Check sheet for the modelled part. Datum: model origin and axes. Units: mm. A direction names the side the tool comes from. Coordinates: 2 decimals unless noted, no trailing zeros. Loops run counter-clockwise (first coordinate to the right, second up) from the corner with the lowest first, then second, coordinate; pieces in that order, holes last. Notation, with made-up numbers: M 22,21.25 L 76,21.25 A35 ccw 76,57.25 Z; hole C 74.5,19.5 d5. An arc over 180 degrees is marked long. Return JSON: item names as keys, results as strings.
from build123d import *

# Parameters (mm, degrees)
F0_W     = 914.4
F0_H     = 914.4
F0_W_2   = 254
F0_H_2   = 889
F0_W_3   = 38.1
F1_DEPTH = 25.4


with BuildPart() as f1:
    # F0 (on Top) → F1 (new body)
    with BuildSketch(Plane.XY):
        with Locations((34.239113, 103.026486)):
            Rectangle(F0_W, F0_H)
        with Locations((-283.260887, 103.026486)):
            Rectangle(F0_W_2, F0_H_2, mode=Mode.SUBTRACT)
        with Locations((-124.510887, 103.026486)):
            Rectangle(F0_W_3, F0_H_2, mode=Mode.SUBTRACT)
        with Locations((34.239113, 103.026486)):
            Rectangle(F0_W_2, F0_H_2, mode=Mode.SUBTRACT)
        with Locations((192.989113, 103.026486)):
            Rectangle(F0_W_3, F0_H_2, mode=Mode.SUBTRACT)
        with Locations((351.739113, 103.026486)):
            Rectangle(F0_W_2, F0_H_2, mode=Mode.SUBTRACT)
    extrude(amount=F1_DEPTH)


solid = f1.part
1) Section check A-A on x = -79. Record the cut outline in (y, z), then the cut area to 3 significant figures.
Answers:
{"outline": "M -354.17,0 L -341.47,0 L -341.47,25.4 L -354.17,25.4 Z; M 547.53,0 L 560.23,0 L 560.23,25.4 L 547.53,25.4 Z", "area": "645 mm²"}
2) Set-up check for faces 5 (the face through (32, -341.474, 13)), 6 (the face through (-103, 105, 0)): record each of +Z, -Z, +X, -X, +Y, -Y from which the full face is reachable in a straight line by a thin tool's end or side.
Answers:
{"face 5": "+Z, -Z", "face 6": "-Z, +X, -X, +Y, -Y"}
3) Draft check along Y on faces 1 (the face through (-156.261, 97, 13)), 2 (the face through (28, -354.174, 13)), 3 (the face through (-422.961, 97, 13)), 4 (the face through (-143.561, 97, 13)). Enter one of: +Y half, -Y half, draft (parallel to the pull), parting line (faces both ways), or undercut.
Answers:
{"face 1": "undercut", "face 2": "-Y half", "face 3": "draft", "face 4": "undercut"}
4) Section check B-B on y = -197.5. Record the cut outline in (x, z), then the cut area to 3 significant figures.
Answers:
{"outline": "M -422.96,0 L -410.26,0 L -410.26,25.4 L -422.96,25.4 Z; M -156.26,0 L -143.56,0 L -143.56,25.4 L -156.26,25.4 Z; M -105.46,0 L -92.76,0 L -92.76,25.4 L -105.46,25.4 Z; M 161.24,0 L 173.94,0 L 173.94,25.4 L 161.24,25.4 Z; M 212.04,0 L 224.74,0 L 224.74,25.4 L 212.04,25.4 Z; M 478.74,0 L 491.44,0 L 491.44,25.4 L 478.74,25.4 Z", "area": "1,940 mm²"}
5) Scan lines: line 1 along X through (y, z) = (454, 5.5); line 2 along Y through (x, z) = (324, 10.25). Record each from-to range of solid material in increasing order. Write a range as [from, to].
Answers:
{"line 1": "[-422.96, -410.26], [-156.26, -143.56], [-105.46, -92.76], [161.24, 173.94], [212.04, 224.74], [478.74, 491.44]", "line 2": "[-354.17, -341.47], [547.53, 560.23]"}
6) Section check C-C on z = 9.75. Record the cut outline in (x, y), then the cut area to 3 significant figures.
Answers:
{"outline": "M -422.96,-354.17 L 491.44,-354.17 L 491.44,560.23 L -422.96,560.23 Z; hole M -410.26,-341.47 L -156.26,-341.47 L -156.26,547.53 L -410.26,547.53 Z; hole M -143.56,-341.47 L -105.46,-341.47 L -105.46,547.53 L -143.56,547.53 Z; hole M -92.76,-341.47 L 161.24,-341.47 L 161.24,547.53 L -92.76,547.53 Z; hole M 173.94,-341.47 L 212.04,-341.47 L 212.04,547.53 L 173.94,547.53 Z; hole M 224.74,-341.47 L 478.74,-341.47 L 478.74,547.53 L 224.74,547.53 Z", "area": "91,000 mm²"}
